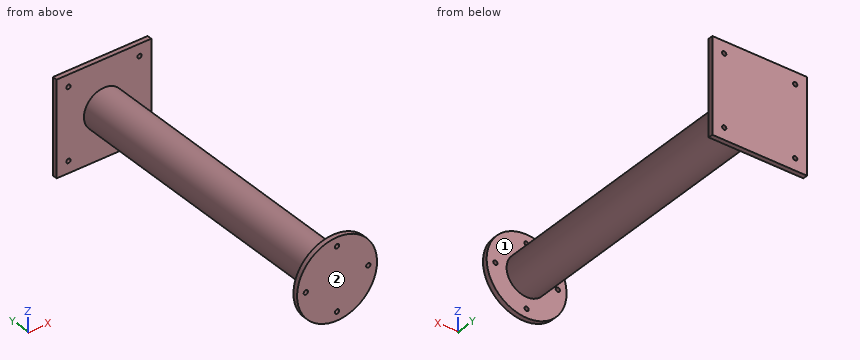
```python
from build123d import *

# Parameters (mm, degrees)
SKETCH1_R           = 84.5
SKETCH1_R_2         = 4.5
BOSS_EXTRUDE4_DEPTH = 10
SKETCH2_R           = 42.25
BOSS_EXTRUDE5_DEPTH = 630
SKETCH4_W           = 200
SKETCH4_H           = 200
BOSS_EXTRUDE6_DEPTH = 10
CUT_EXTRUDE1_DEPTH  = 666.206734783


with BuildPart() as part:
    # Sketch1 → Boss-Extrude4 (new body)
    with BuildSketch(Plane(origin=(0, 0, 0), x_dir=(1, 0, 0), z_dir=(0, 1, 0))):
        with Locations(Location((0, 0, 0), (0, 0, 270))):
            Circle(SKETCH1_R)
        with Locations(Location((0, -66, 0), (0, 0, 270))):
            Circle(SKETCH1_R_2, mode=Mode.SUBTRACT)
        with Locations(Location((66, 0, 0), (0, 0, 270))):
            Circle(SKETCH1_R_2, mode=Mode.SUBTRACT)
        with Locations(Location((-66, 0, 0), (0, 0, 270))):
            Circle(SKETCH1_R_2, mode=Mode.SUBTRACT)
        with Locations(Location((0, 66, 0), (0, 0, 270))):
            Circle(SKETCH1_R_2, mode=Mode.SUBTRACT)
    extrude(amount=BOSS_EXTRUDE4_DEPTH)

    # Sketch2 → Boss-Extrude5 (add)
    with BuildSketch(Plane(origin=(0, 10, 0), x_dir=(1, 0, 0), z_dir=(0, 1, 0))):
        with Locations(Location((0, 0, 0), (0, 0, 270))):
            Circle(SKETCH2_R)
    extrude(amount=BOSS_EXTRUDE5_DEPTH)

    # Sketch4 → Boss-Extrude6 (add)
    with BuildSketch(Plane(origin=(0, 640, 0), x_dir=(1, 0, 0), z_dir=(0, 1, 0))):
        Rectangle(SKETCH4_W, SKETCH4_H)
    extrude(amount=BOSS_EXTRUDE6_DEPTH)

    # Sketch5 → Cut-Extrude1 (cut, through all)
    with BuildSketch(Plane(origin=(0, 650, 0), x_dir=(1, 0, 0), z_dir=(0, 1, 0))):
        with BuildLine():
            Line((-75, -70.5), (-75, -75))
            Line((-75, -75), (-70.5, -75))
            ThreePointArc((-70.5, -75), (-71.818019485, -71.818019485), (-75, -70.5))
        make_face()
        with BuildLine():
            Line((-70.5, -75), (-75, -75))
            Line((-75, -75), (-75, -70.5))
            ThreePointArc((-75, -70.5), (-78.181980515, -78.181980515), (-70.5, -75))
        make_face()
        with BuildLine():
            ThreePointArc((-70.5, 75), (-78.181980515, 78.181980515), (-75, 70.5))
            Line((-75, 70.5), (-75, 75))
            Line((-75, 75), (-70.5, 75))
        make_face()
        with BuildLine():
            Line((-75, 75), (-75, 70.5))
            ThreePointArc((-75, 70.5), (-71.818019485, 71.818019485), (-70.5, 75))
            Line((-70.5, 75), (-75, 75))
        make_face()
        with BuildLine():
            ThreePointArc((70.5, 75), (71.818019485, 71.818019485), (75, 70.5))
            Line((75, 70.5), (75, 75))
            Line((75, 75), (70.5, 75))
        make_face()
        with BuildLine():
            Line((75, 75), (75, 70.5))
            ThreePointArc((75, 70.5), (78.181980515, 71.818019485), (79.5, 75))
            ThreePointArc((79.5, 75), (75, 79.5), (70.5, 75))
            Line((70.5, 75), (75, 75))
        make_face()
        with BuildLine():
            ThreePointArc((75, -70.5), (71.818019485, -71.818019485), (70.5, -75))
            Line((70.5, -75), (75, -75))
            Line((75, -75), (75, -70.5))
        make_face()
        with BuildLine():
            Line((75, -75), (70.5, -75))
            ThreePointArc((70.5, -75), (75, -79.5), (79.5, -75))
            ThreePointArc((79.5, -75), (78.181980515, -71.818019485), (75, -70.5))
            Line((75, -70.5), (75, -75))
        make_face()
    extrude(amount=-CUT_EXTRUDE1_DEPTH, mode=Mode.SUBTRACT)


solid = part.part
```
Read the model definition and answer for the solid it produces. Units are mm, in the model's axes. Face numbers are marked on the shaded views. A direction names the side the tool comes from. Coordinates: 2 decimals unless noted, no trailing zeros. Order: outer loops, then holes, each group sorted by start corner. A loop starts at its lowest first (then second) coordinate and runs counter-clockwise, first axis right, second up. Notation, with made-up numbers: (67, 83.5) - (71, 83.5) arc R19 cw to (71, 97.5) - close; hole circle Ø4 at (-2.5, -12). An arc over 180 degrees is marked (long way). Answer as a JSON object with one key per item and string values. Group by question number.
Item 1: Section A-A (y = 86.5) is taken. Give the vertices of the cut face in (x, z), plus the area to 3 significant figures.
Item 2: Section B-B (x = -27.5) is taken. Give the vertices of the cut face in (y, z), plus the area to 3 significant figures.
Item 3: Consider probe 1 along X at (y, z) = (643, -75); probe 2 along X at (y, z) = (3.75, 0). Determine where each line is inside the solid, lowest interval first. Write a range as from..to.
Item 4: A tool of negligible diameter and unlimited length cuts with its end or side. For the marked faces 1 and 2, from which of +Z, -Z, +X, -X, +Y, -Y can it reach the whole face along a straight path? Write none if from no direction.
Item 5: Flat-ended cylindrical pins translate along their axes: P1, Ø1, axis at x = -9, y = 512.5, coming from the +Z side; P2, Ø8, axis at x = -66, z = 0, coming from the -Y side; P3, Ø5, axis at y = 345, z = 31.5, coming from the +X side. Find the tip coordinate at first contact, or state that the pin passes through.
Results are:
{
 "1": {"outline": "circle Ø84.5 at (0, 0)", "area": "5,610 mm^2"},
 "2": {"outline": "(0, -79.9) - (10, -79.9) - (10, -32.08) - (640, -32.08) - (640, -100) - (650, -100) - (650, 100) - (640, 100) - (640, 32.08) - (10, 32.08) - (10, 79.9) - (0, 79.9) - close", "area": "44,000 mm^2"},
 "3": {"probe 1": "x = -100..-79.5, -70.5..70.5, 79.5..100", "probe 2": "x = -84.5..-70.5, -61.5..61.5, 70.5..84.5"},
 "4": {"face 1": "none", "face 2": "+Z, -Z, +X, -X, -Y"},
 "5": {"P1": "stops at z = 41.39", "P2": "stops at y = 640", "P3": "stops at x = 30.73"}
}
